Verification items for this drawing (mm, ordinates from the low corner). A direction names the side the tool comes from. Round coordinates to 2 decimals unless told otherwise and drop trailing zeros. Loops run counter-clockwise (first coordinate to the right, second up) from the corner with the lowest first, then second, coordinate; pieces in that order, holes last. Notation, with made-up numbers: (15, -36) -> (70, -36) arc R16 ccw to (70, -17) -> close; hole circle Ø2 at (23.25, 0.5). An arc over 180 degrees is marked (long way). One line per question, with ' | ' between items.
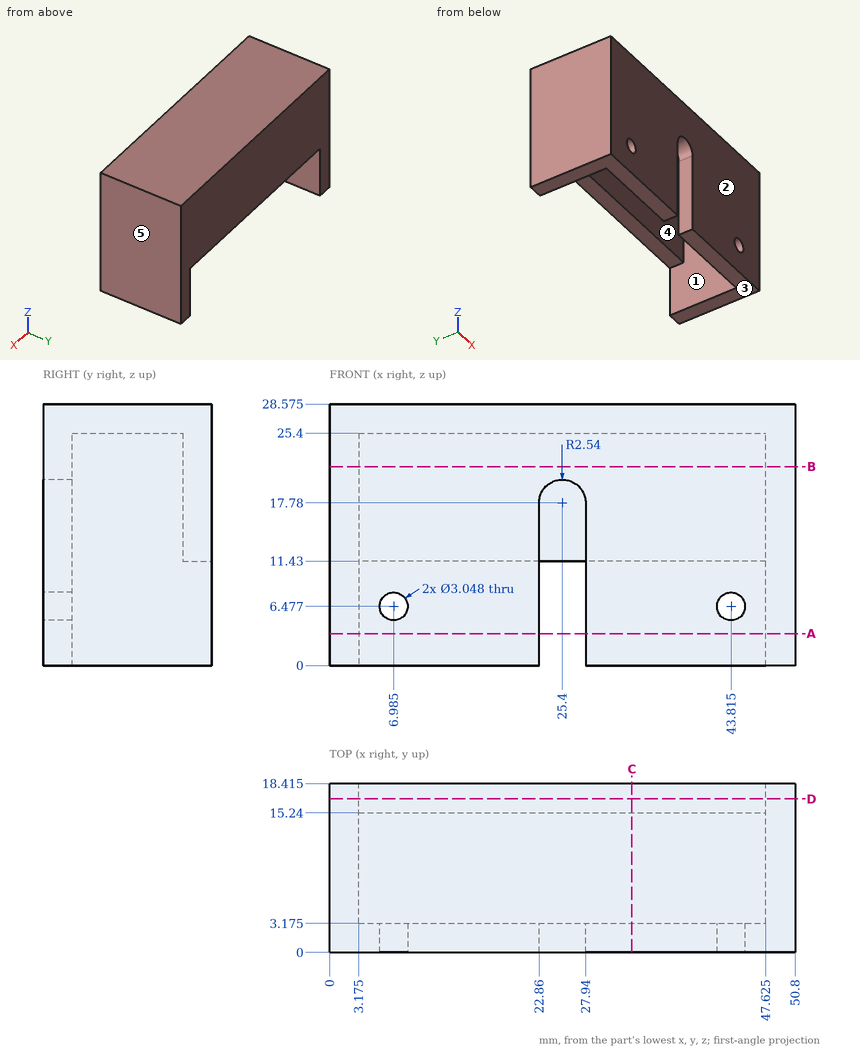
(1) Go/stop test with flat-tipped pins: pin 1 (2.5 mm diameter, centred on x = 23, y = 16.5, fed in from -Z); pin 2 (1.8 mm diameter, centred on x = 6.985, z = 6.477, fed in from -Y). Record where each tip stops, or that it passes through.
Answer:
pin 1: stops at z = 11.43 | pin 2: passes through
(2) Sectioned sample at A-A, the plane z = 3.5. Record the cut outline in (x, y) (3 decimals), and give its area (3 significant figures).
Answer:
outline: (0, 0) -> (22.86, 0) -> (22.86, 3.175) -> (3.175, 3.175) -> (3.175, 18.415) -> (0, 18.415) -> close; (27.94, 0) -> (50.8, 0) -> (50.8, 18.415) -> (47.625, 18.415) -> (47.625, 3.175) -> (27.94, 3.175) -> close | area: 242 mm2
(3) Sectioned sample at D-D, the plane y = 16.75. Record the cut outline in (x, z) (3 decimals), and give its area (3 significant figures).
Answer:
outline: (0, 0) -> (3.175, 0) -> (3.175, 11.43) -> (47.625, 11.43) -> (47.625, 0) -> (50.8, 0) -> (50.8, 28.575) -> (0, 28.575) -> close | area: 944 mm2
(4) Set-up check for the marked faces 4 and 5: record each of +Z, -Z, +X, -X, +Y, -Y from which the full face is reachable in a straight line by a thin tool's end or side.
Answer:
face 4: -Z | face 5: +Z, -Z, +X, +Y, -Y
(5) Sectioned sample at B-B, the plane z = 21.75. Record the cut outline in (x, y) (3 decimals), and give its area (3 significant figures).
Answer:
outline: (0, 0) -> (50.8, 0) -> (50.8, 18.415) -> (0, 18.415) -> close; hole (3.175, 3.175) -> (47.625, 3.175) -> (47.625, 15.24) -> (3.175, 15.24) -> close | area: 399 mm2
(6) Sectioned sample at C-C, the plane x = 33. Record the cut outline in (y, z) (3 decimals).
Answer:
outline: (0, 0) -> (3.175, 0) -> (3.175, 25.4) -> (15.24, 25.4) -> (15.24, 11.43) -> (18.415, 11.43) -> (18.415, 28.575) -> (0, 28.575) -> close
(7) Scan lines: probe 1 along X at (y, z) = (14.75, 22.25) (3 decimals); probe 2 along Y at (x, z) = (41.5, 17.25) (3 decimals); probe 3 along X at (y, z) = (2.5, 5.5). Record each from-to range of solid material in increasing order.
Answer:
probe 1: x = 0 to 3.175, 47.625 to 50.8 | probe 2: y = 0 to 3.175, 15.24 to 18.415 | probe 3: x = 0 to 5.82, 8.15 to 22.86, 27.94 to 42.65, 44.98 to 50.8
(8) Mould release check, pull along Y, two halves, no side actions. Record for the marked faces 1, 2 and 3: +Y half, -Y half, draft (parallel to the pull), parting line (faces both ways), or undercut.
Answer:
face 1: undercut | face 2: -Y half | face 3: draft
